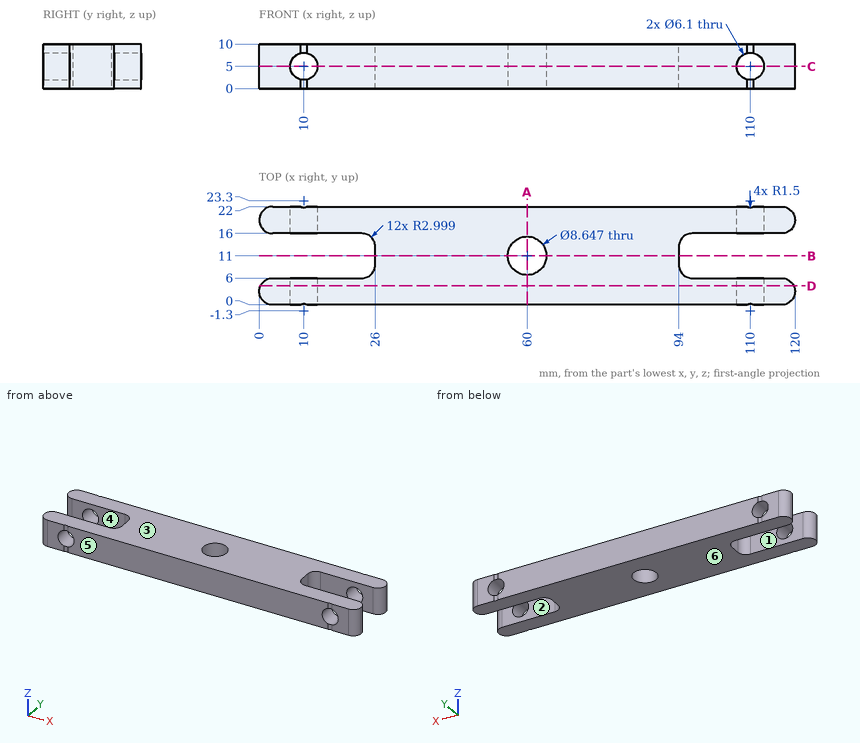
Answer from the drawing. Dimensions are ordinates in mm from the lowest x, y and z of the part. A direction names the side the tool comes from. Round coordinates to 2 decimals unless told otherwise and drop trailing zeros. Loops run counter-clockwise (first coordinate to the right, second up) from the corner with the lowest first, then second, coordinate; pieces in that order, holes last.
Q1. Section A-A on x = 60 is taken. Write down the section's boundary in (y, z).
Q2. Section D-D on y = 4.25 is taken. Write down the section's boundary in (x, z).
Q3. Which of the six approach directions +Z, -Z, +X, -X, +Y, -Y give full straight-line access (tool end or side, diameter ignored) to the marked faces 1, 2 and 3?
Q4. Each of these flat-tipped pins is pushed along its axis until it touches: pin 1 (3 mm diameter, centred on y = 11, z = 4.5, fed in from -X); pin 2 (4 mm diameter, centred on y = 10.5, z = 2.5, fed in from +X); pin 3 (6 mm diameter, centred on y = 7.5, z = 5.5, fed in from -X); pin 4 (5 mm diameter, centred on x = 110, z = 5, fed in from -Y). Where does it stop, or does it pass through?
Q5. Consider probe 1 along Y at (x, z) = (105, 7.5); probe 2 along X at (y, z) = (11, 3.5); probe 3 along Z at (x, y) = (110, 4.75). Determine where each line is inside the solid, lowest interval first.
Q6. Section B-B on y = 11 is taken. Write down the section's boundary in (x, z).
Q7. Section C-C on z = 5 is taken. Give the number of separate pieces and of enclosed holes in the cut face, and give its area (3 significant figures).
Q8. Determine the mould class of the marked faces 4, 5 and 6 for opening direction Y: released by +Y, released by -Y, zero draft, split by the parting line, or undercut.
Output:
1. outline: (0, 0) - (6.68, 0) - (6.68, 10) - (0, 10) - close; (15.32, 0) - (22, 0) - (22, 10) - (15.32, 10) - close
2. outline: (0.27, 0) - (119.73, 0) - (119.73, 10) - (0.27, 10) - close; hole circle Ø6.1 at (10, 5); hole circle Ø6.1 at (110, 5)
3. face 1: +Z, -Z, -X
3. face 2: +Z, -Z, +X
3. face 3: +Z, +X, -X, +Y, -Y
4. pin 1: stops at x = 26
4. pin 2: stops at x = 94.04
4. pin 3: stops at x = 0.4
4. pin 4: passes through
5. probe 1: y = 0 to 6, 16 to 22
5. probe 2: x = 26 to 55.68, 64.32 to 94
5. probe 3: z = 0 to 1.95, 8.05 to 10
6. outline: (26, 0) - (55.68, 0) - (55.68, 10) - (26, 10) - close; (64.32, 0) - (94, 0) - (94, 10) - (64.32, 10) - close
7. separate pieces: 5
7. enclosed holes: 1
7. area: 1,910 mm2
8. face 4: undercut
8. face 5: released by -Y
8. face 6: zero draft
